Source: CAD feature listing. Evaluate the final solid. Frame: model axes, mm. Face numbers are marked on the shaded views. A direction names the side the tool comes from. Give positions to 0.01 mm unless a question says otherwise; leave off trailing zeros. Write each loop counter-clockwise with the first axis right and the second up, starting at its lowest first coordinate (ties: lowest second). Pieces come first, ordered by that corner, then holes. Notation, with made-up numbers: (71.5, -29) -> (113.5, -29) arc R14 ccw to (113.5, -9) -> close; hole circle Ø8 at (55.25, 43). An arc over 180 degrees is marked (long way). Answer as a JSON object with one key per item and string values. Group by question number.
Item 1: Ray query, probe 1 along X at (y, z) = (7.5, -15); probe 2 along X at (y, z) = (7.75, -19); probe 3 along Z at (x, y) = (-5.75, 5.5). Return the intervals inside material, ascending. Write a range as from..to.
Item 2: Section query D-D on z = 6. Return the cut outline in (x, y).
Item 3: Access query for the marked faces 1, 2 and 3. Directions: +Z, -Z, +X, -X, +Y, -Y. A direction counts if a zero-diameter tool reaches every point of the face in a straight line with its end or side. Return the directions, or none.
Item 4: Section query A-A on y = 4.5. Return the cut outline in (x, z), plus the area to 3 significant figures.
Item 5: First-contact query: pin 1 Ø1 at (y, z) = (6.5, -18) entering from -X; pin 2 Ø4 at (x, z) = (4, -16.5) entering from +Y. Flat tips, straight axial feed; report the tip coordinate or a pass-through.
Item 6: Section query C-C on y = 7.5. Return the cut outline in (x, z), plus the area to 3 significant figures.
Item 7: Section query B-B on z = -21. Return the cut outline in (x, y).
Autodesk Inventor part; units mm, degrees
ref_plane "YZ Plane" through (0, 0, 0) normal (1, 0, 0) x (0, 1, 0)
ref_plane "XZ Plane" through (0, 0, 0) normal (0, 1, 0) x (-1, 0, 0)
ref_plane "XY Plane" through (0, 0, 0) normal (0, 0, 1) x (1, 0, 0)
sketch "Эскиз1" plane through (0, 0, 0) normal (0, 1, 0) x (-1, 0, 0)
  line L0 (-7.25, -10) -> (7.25, -10)
  line L1 (7.25, -10) -> (7.25, 4)
  line L2 (1.25, 10) -> (-1.25, 10)
  line L3 (-7.25, 4) -> (-7.25, -10)
  line L4 (-7.25, -10) -> (7.25, 10) construction
  line L5 (7.25, -10) -> (-7.25, 10) construction
  arc A0 (7.25, 4) -> (1.25, 10) centre (1.25, 4) ccw
  arc A1 (-1.25, 10) -> (-7.25, 4) centre (-1.25, 4) ccw
  line L6 (0, -10) -> (5, -10)
  point P0 (0, 0)
  dimension "d0" = 14.5
  dimension "d1" = 20
  dimension "d2" = 6
  dimension "d3" = 6
extrude "Выдавливание1" add sketch "Эскиз1" along normal blind 9
sketch "Эскиз3" plane through (7.25, 0, -10) normal (0, 0, -1) x (-1, 0, 0)
  line L0 (0, 0) -> (0, 9)
  line L1 (14.5, 0) -> (8.5, 0)
  line L2 (0, 9) -> (14.5, 9)
  line L3 (14.5, 9) -> (14.5, 0)
  line L4 (14.5, 0) -> (0, 0)
  line L5 (0, 0) -> (0, 9)
  circle A0 centre (7, 4.5) radius 4.5
  point P0 (7.25, 0)
  dimension "d11" = 9
  dimension "d12" = 4.5
extrude "Выдавливание3" add sketch "Эскиз3" along normal blind 13 contours A0
properties part number "moroshenka"
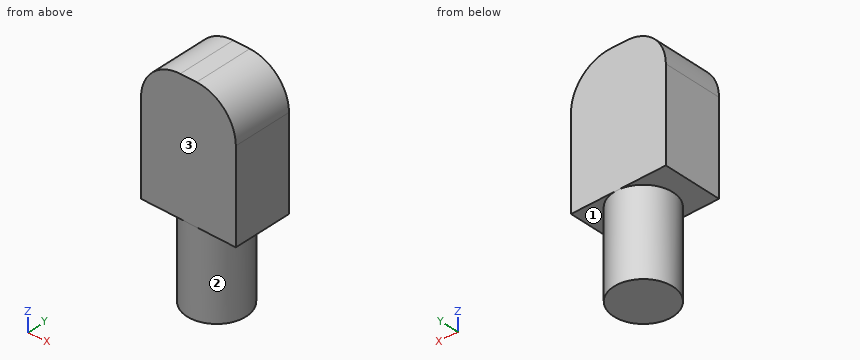
Worked answers:
{
 "1": {"probe 1": "-3.1..3.6", "probe 2": "-2.86..3.36", "probe 3": "-10..7.97"},
 "2": {"outline": "(-6.91, 0) -> (6.91, 0) -> (6.91, 9) -> (-6.91, 9) -> close"},
 "3": {"face 1": "-Z, +X", "face 2": "-Z", "face 3": "+Z, -Z, +X, -X, -Y"},
 "4": {"outline": "(-7.25, -10) -> (-4.25, -10) -> (-4.25, -23) -> (4.75, -23) -> (4.75, -10) -> (7.25, -10) -> (7.25, 4) arc R6 ccw to (1.25, 10) -> (-1.25, 10) arc R6 ccw to (-7.25, 4) -> close", "area": "392 mm^2"},
 "5": {"pin 1": "x = -3.99", "pin 2": "y = 8.65"},
 "6": {"outline": "(-7.25, -10) -> (-3.1, -10) -> (-3.1, -23) -> (3.6, -23) -> (3.6, -10) -> (7.25, -10) -> (7.25, 4) arc R6 ccw to (1.25, 10) -> (-1.25, 10) arc R6 ccw to (-7.25, 4) -> close", "area": "362 mm^2"},
 "7": {"outline": "circle Ø9 at (0.25, 4.5)"}
}
